Print and shaded views of the part. All mm, measured from the part's lowest x, y and z. Round coordinates to 2 decimals unless told otherwise and drop trailing zeros. Loops run counter-clockwise (first coordinate to the right, second up) from the corner with the lowest first, then second, coordinate; pieces in that order, holes last. Notation, with made-up numbers: (88.25, -25.75) - (132.25, -25.75) arc R13 ccw to (132.25, -10.75) - close; hole circle Ø1 at (55, 55). An arc over 180 degrees is marked (long way). Answer as a JSON object with one key per item and string values.
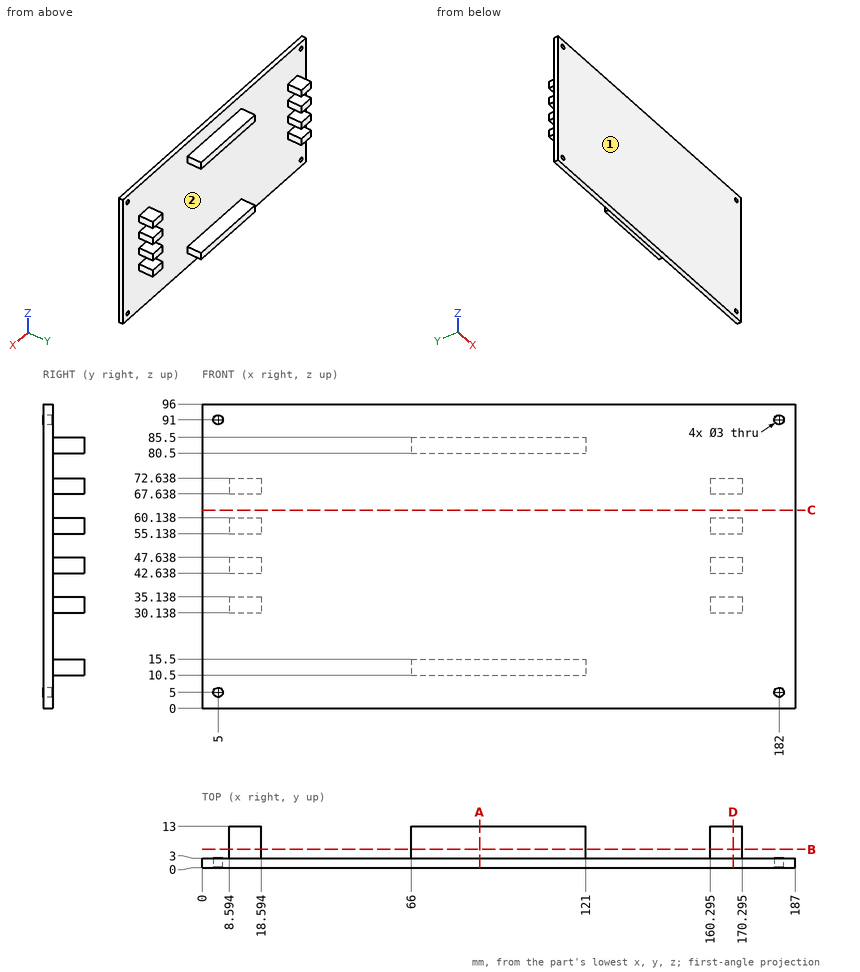
1) Slice it at C-C on z = 62.5. List the corners of the cut face in (x, y), then the cut area to 3 significant figures.
Values follow:
{"outline": "(0, 0) - (187, 0) - (187, 3) - (0, 3) - close", "area": "561 mm²"}
2) Drop flat-ended pins along their axis: P1, Ø4, axis at x = 89, z = 77, coming from the +Y side; P2, Ø5.5, axis at y = 7.5, z = 33.5, coming from the +X side (3 decimals); P3, Ø2, axis at y = 6, z = 56, coming from the -X side. Give the stop position or say it passes through.
Values follow:
{"P1": "y = 3", "P2": "x = 170.295", "P3": "x = 8.59"}
3) Slice it at A-A on x = 87.5. List the corners of the cut face in (y, z), then the cut area to 3 significant figures.
Values follow:
{"outline": "(0, 0) - (3, 0) - (3, 10.5) - (13, 10.5) - (13, 15.5) - (3, 15.5) - (3, 80.5) - (13, 80.5) - (13, 85.5) - (3, 85.5) - (3, 96) - (0, 96) - close", "area": "388 mm²"}
4) Slice it at D-D on x = 167.5. List the corners of the cut face in (y, z).
Values follow:
{"outline": "(0, 0) - (3, 0) - (3, 30.14) - (13, 30.14) - (13, 35.14) - (3, 35.14) - (3, 42.64) - (13, 42.64) - (13, 47.64) - (3, 47.64) - (3, 55.14) - (13, 55.14) - (13, 60.14) - (3, 60.14) - (3, 67.64) - (13, 67.64) - (13, 72.64) - (3, 72.64) - (3, 96) - (0, 96) - close"}
5) Two-plate mould, pull along Z, no slides. Class the marked faces 1 and 2: pulls with the +Z half, pulls with the -Z half, needs draft (parallel to the pull), parting line crosses it, or undercut.
Values follow:
{"face 1": "needs draft", "face 2": "undercut"}
6) Slice it at B-B on y = 5.75. Count the separate pieces of the cut face and the enclosed holes in it, then the cut area to 3 significant figures.
Values follow:
{"separate pieces": "10", "enclosed holes": "0", "area": "950 mm²"}
7) Probe probe 1 along Z at (x, y) = (182, 2); probe 2 along X at (y, z) = (2.2, 91); probe 3 along X at (y, z) = (5.25, 60) (1 decimal). List the from-to ranges inside material, lowest first.
Values follow:
{"probe 1": "0 to 3.5, 6.5 to 89.5, 92.5 to 96", "probe 2": "0 to 3.5, 6.5 to 180.5, 183.5 to 187", "probe 3": "8.6 to 18.6, 160.3 to 170.3"}
